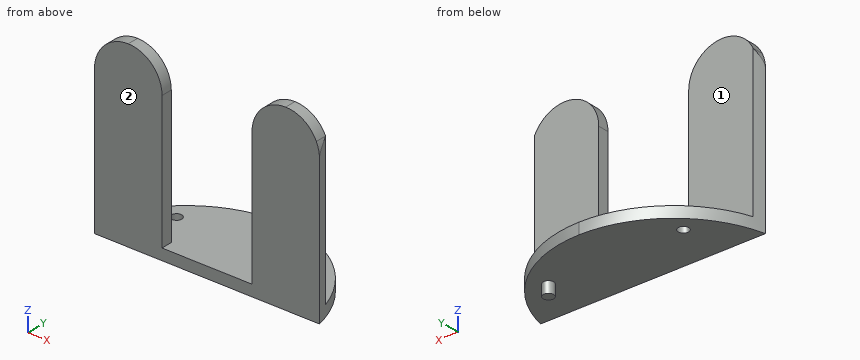
```python
from build123d import *

# Parameters (mm, degrees)
BOSS_EXTRUDE1_DEPTH = 63.5
SKETCH3_R           = 1.5
CUT_EXTRUDE1_DEPTH  = 86.194189943
SKETCH3_3_R         = 1.5
BOSS_EXTRUDE2_DEPTH = 3.175
CUT_EXTRUDE2_DEPTH  = 86.194189943
CUT_EXTRUDE3_DEPTH  = 3.175


with BuildPart() as part:
    # Sketch2 → Boss-Extrude1 (new body)
    with BuildSketch(Plane(origin=(0, 0, 0), x_dir=(0, 0, -1), z_dir=(1, 0, 0))):
        Polygon((-50.8, 0), (0, 0), (0, 25.4), (-3.175, 25.4), (-3.175, 3.175), (-50.8, 3.175), align=None)
    extrude(amount=BOSS_EXTRUDE1_DEPTH)

    # Sketch3 → Cut-Extrude1 (cut, through all)
    with BuildSketch(Plane(origin=(0, 0, 0), x_dir=(-1, 0, 0), z_dir=(0, 0, -1))):
        with Locations(Location((-12.7, 12.7, 0), (0, 0, 90))):
            Circle(SKETCH3_R)
    extrude(amount=-CUT_EXTRUDE1_DEPTH, mode=Mode.SUBTRACT)

    # Sketch3_3 → Boss-Extrude2 (add)
    with BuildSketch(Plane(origin=(0, 0, 0), x_dir=(-1, 0, 0), z_dir=(0, 0, -1))):
        with Locations(Location((-50.8, 12.7, 0), (0, 0, 180))):
            Circle(SKETCH3_3_R)
    extrude(amount=BOSS_EXTRUDE2_DEPTH)

    # Sketch4 → Cut-Extrude2 (cut, through all)
    with BuildSketch(Plane(origin=(0, 0, 0), x_dir=(-1, 0, 0), z_dir=(0, 0, -1))):
        with BuildLine():
            Line((-63.5, 25.4), (-63.5, 0))
            ThreePointArc((-63.5, 0), (-52.079919454, 18.268649317), (-31.75, 25.4))
            Line((-31.75, 25.4), (-63.5, 25.4))
        make_face()
        with BuildLine():
            ThreePointArc((-31.75, 25.4), (-11.420080546, 18.268649317), (0, 0))
            Line((0, 0), (0, 25.4))
            Line((0, 25.4), (-31.75, 25.4))
        make_face()
    extrude(amount=-CUT_EXTRUDE2_DEPTH, mode=Mode.SUBTRACT)

    # Sketch5 → Cut-Extrude3 (cut)
    with BuildSketch(Plane(origin=(0, 3.175, 0), x_dir=(1, 0, 0), z_dir=(0, 1, 0))):
        with BuildLine():
            Line((44.45, -3.175), (19.05, -3.175))
            Line((19.05, -3.175), (19.05, -41.275))
            ThreePointArc((19.05, -41.275), (16.260192091, -48.010192091), (9.525, -50.8))
            Line((9.525, -50.8), (53.975, -50.8))
            ThreePointArc((53.975, -50.8), (47.239807909, -48.010192091), (44.45, -41.275))
            Line((44.45, -41.275), (44.45, -3.175))
        make_face()
        with BuildLine():
            ThreePointArc((9.525, -50.8), (4.400279527, -49.303876949), (0.885472424, -45.285509726))
            Line((0.885472424, -45.285509726), (0.885472424, -50.8))
            Line((0.885472424, -50.8), (9.525, -50.8))
        make_face()
        with BuildLine():
            ThreePointArc((0.885472424, -45.285509726), (0.224002065, -43.328548738), (0, -41.275))
            Line((0, -41.275), (0, -50.8))
            Line((0, -50.8), (0.885472424, -50.8))
            Line((0.885472424, -50.8), (0.885472424, -45.285509726))
        make_face()
        with BuildLine():
            ThreePointArc((62.614527576, -45.285509726), (59.099720473, -49.303876949), (53.975, -50.8))
            Line((53.975, -50.8), (62.614527576, -50.8))
            Line((62.614527576, -50.8), (62.614527576, -45.285509726))
        make_face()
        with BuildLine():
            ThreePointArc((63.5, -41.275), (63.275997935, -43.328548738), (62.614527576, -45.285509726))
            Line((62.614527576, -45.285509726), (62.614527576, -50.8))
            Line((62.614527576, -50.8), (63.5, -50.8))
            Line((63.5, -50.8), (63.5, -41.275))
        make_face()
    extrude(amount=-CUT_EXTRUDE3_DEPTH, mode=Mode.SUBTRACT)


solid = part.part
```
Verification items for the finished model (mm, model axes). Face numbers are marked on the shaded views. A direction names the side the tool comes from. Give positions to 0.01 mm unless a question says otherwise; leave off trailing zeros. Order: outer loops, then holes, each group sorted by start corner. A loop starts at its lowest first (then second) coordinate and runs counter-clockwise, first axis right, second up. Notation, with made-up numbers: (19, 68) - (61, 68) arc R11 ccw to (61, 82) - close; hole circle Ø4 at (39, 21). An arc over 180 degrees is marked (long way). Answer as CSV lines item,"result". Start each with the question number.
Item 1: Material ranges on L1, parallel to Z at x = 41, y = 10.75 (3 decimals); L2, parallel to X at y = 12.7, z = 2.3, recorded low to high.
Item 2: Section check C-C, the plane x = 12.7. Record the boundary of the cut face in (y, z) (3 decimals), plus the area to 3 significant figures.
Item 3: Section check B-B, the plane y = 12.7. Record the boundary of the cut face in (x, z) (3 decimals).
Item 4: Gauge pin test, flat ends, axial feed: pin 1 (3 mm diameter, centred on x = 41.5, y = 6.5, fed in from -Z); pin 2 (20 mm diameter, centred on x = 14.5, z = 38, fed in from +Y) (3 decimals); pin 3 (8 mm diameter, centred on x = 43.5, y = 18, fed in from +Z) (3 decimals); pin 4 (12 mm diameter, centred on y = 15.5, z = 13, fed in from +X). Record the tip position at first contact, or that the pin passes through.
Item 5: Access from +Z, -Z, +X, -X, +Y, -Y to the whole of each face (thin tool, end or side, straight path). Record for the marked faces 1 and 2.
Filled in:
1,L1,"0 to 3.175"
1,L2,"5.96 to 11.2, 14.2 to 57.54"
2,outline,"(0, 0) - (11.2, 0) - (11.2, 3.175) - (3.175, 3.175) - (3.175, 50.255) - (0, 50.255) - close; (14.2, 0) - (19.242, 0) - (19.242, 3.175) - (14.2, 3.175) - close"
2,area,"201 mm^2"
3,outline,"(5.956, 0) - (11.2, 0) - (11.2, 3.175) - (5.956, 3.175) - close; (14.2, 0) - (49.3, 0) - (49.3, -3.175) - (52.3, -3.175) - (52.3, 0) - (57.544, 0) - (57.544, 3.175) - (14.2, 3.175) - close"
4,pin 1,"z = 0"
4,pin 2,"y = 3.175"
4,pin 3,"z = 3.175"
4,pin 4,"through"
5,face 1,"+Z, +X, -X, +Y"
5,face 2,"+Z, -Z, +X, -X, -Y"
